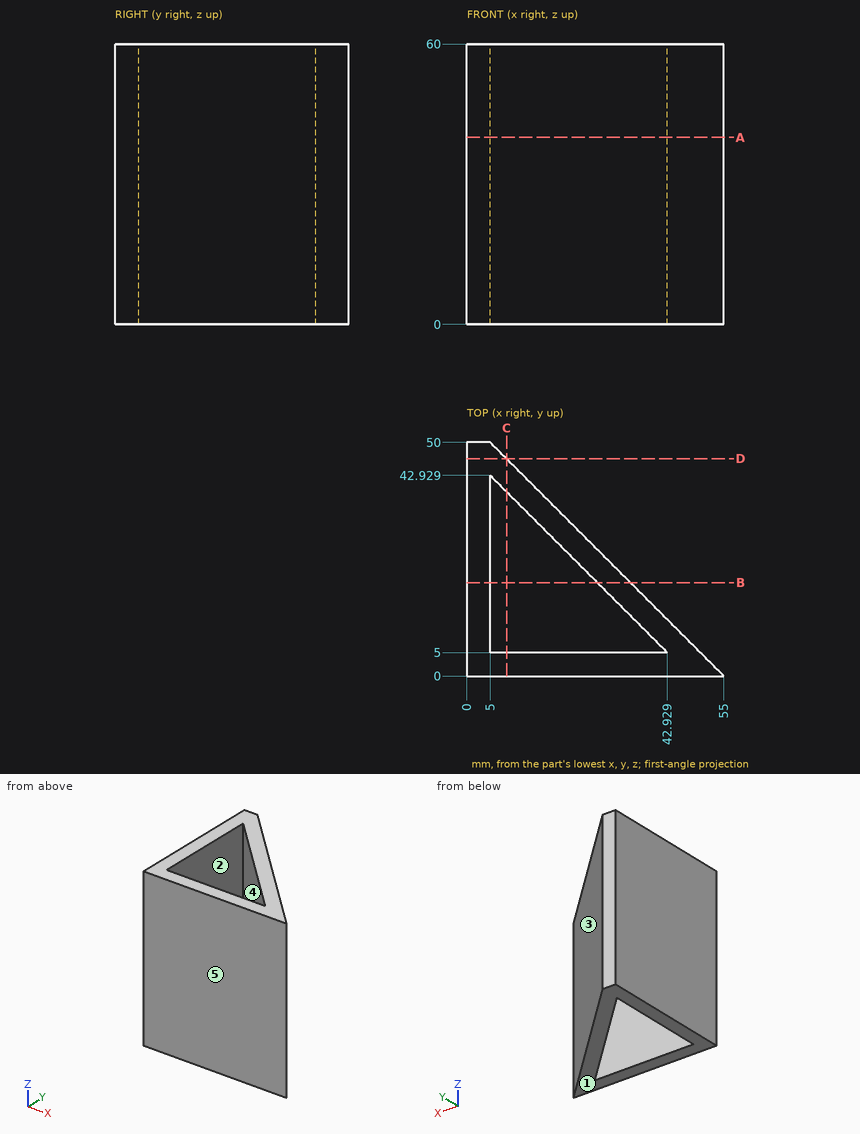
Print and shaded views of the part. All mm, measured from the part's lowest x, y and z. A direction names the side the tool comes from. Round coordinates to 2 decimals unless told otherwise and drop trailing zeros. Order: outer loops, then holes, each group sorted by start corner. A loop starts at its lowest first (then second) coordinate and runs counter-clockwise, first axis right, second up.
Q1. Slice it at C-C (x = 8.5). Write the cut outline in (y, z).
Q2. Slice it at B-B (y = 20). Write the cut outline in (x, z).
Q3. Which spindle directions (+Z, -Z, +X, -X, +Y, -Y) get a long thin tool onto all of the face, cutting with end or side? Do the marked faces 1 and 2. Say none if no direction does.
Q4. Drop flat-ended pins along their axis: pin 1 (1 mm diameter, centred on x = 14.5, z = 36.5, fed in from +Y); pin 2 (10 mm diameter, centred on y = 40.5, z = 38, fed in from +X); pin 3 (1 mm diameter, centred on x = 11, z = 54, fed in from +Y). Give the stop position or say it passes through.
Q5. Two-plate mould, pull along X, no slides. Class the marked faces 3, 4 and 5: pulls with the +X half, pulls with the -X half, needs draft (parallel to the pull), parting line crosses it, or undercut.
Q6. Slice it at A-A (z = 40). Write the cut outline in (x, y), and give its area (3 significant figures).
Q7. Wall check: L1, parallel to X at y = 8.5, z = 18.5; L2, parallel to X at y = 38.5, z = 54; L3, parallel to Y at x = 41, z = 30. Give the ranges that are in metal, low to high.
Q8. Slice it at D-D (y = 46.5). Write the cut outline in (x, z).
Results below:
1. outline: (0, 0) - (5, 0) - (5, 60) - (0, 60) - close; (39.43, 0) - (46.5, 0) - (46.5, 60) - (39.43, 60) - close
2. outline: (0, 0) - (5, 0) - (5, 60) - (0, 60) - close; (27.93, 0) - (35, 0) - (35, 60) - (27.93, 60) - close
3. face 1: -Z, +X, -X, +Y, -Y
3. face 2: +Z, -Z
4. pin 1: stops at y = 41
4. pin 2: stops at x = 19.5
4. pin 3: stops at y = 44.5
5. face 3: pulls with the +X half
5. face 4: undercut
5. face 5: needs draft
6. outline: (0, 0) - (55, 0) - (5, 50) - (0, 50) - close; hole (5, 5) - (42.93, 5) - (5, 42.93) - close
6. area: 781 mm2
7. L1: x = 0 to 5, 39.43 to 46.5
7. L2: x = 0 to 5, 9.43 to 16.5
7. L3: y = 0 to 5, 6.93 to 14
8. outline: (0, 0) - (8.5, 0) - (8.5, 60) - (0, 60) - close
